Build history of the part. All positions in model axes, mm. Face numbers are marked on the shaded views. A direction names the side the tool comes from. Give positions to 0.01 mm unless a question says otherwise; leave off trailing zeros. Order: outer loops, then holes, each group sorted by start corner. A loop starts at its lowest first (then second) coordinate and runs counter-clockwise, first axis right, second up. Notation, with made-up numbers: (39.25, -22) - (70.25, -22) arc R15 ccw to (70.25, 3) - close; hole circle Ø3 at (86, -39). An arc over 180 degrees is marked (long way). Use a Markdown table: item, result.
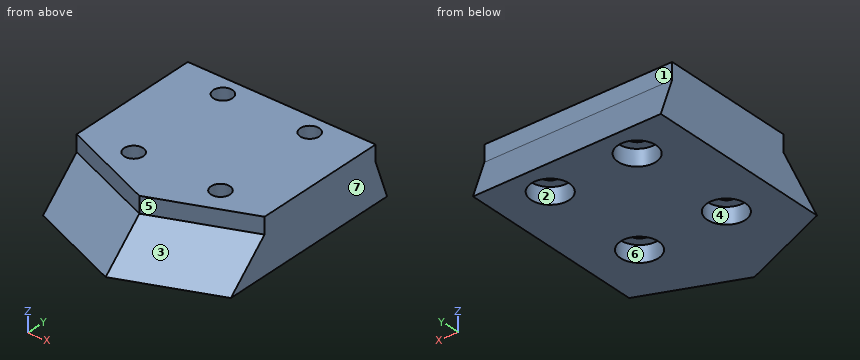
from build123d import *

# Parameters (mm, degrees)
ESBO_O1_W                = 34.6
ESBO_O1_H                = 26
RESSALTO_EXTRUS_O1_DEPTH = 7
ESBO_O10_W               = 34.6
ESBO_O10_H               = 2.5
RESSALTO_EXTRUS_O4_DEPTH = 7
CHANFRO1_SIZE            = 7
CHANFRO2_SIZE2           = 7
CHANFRO2_SIZE            = 2.54779164
RESSALTO_EXTRUS_O5_DEPTH = 3
ESBO_O11_R               = 1.75
CORTE_EXTRUS_O1_DEPTH    = 10
ESBO_O12_R               = 3.5
CORTE_EXTRUS_O2_DEPTH    = 3


with BuildPart() as part:
    # Esboço1 → Ressalto-extrusão1 (new body)
    with BuildSketch(Plane.XY):
        Rectangle(ESBO_O1_W, ESBO_O1_H)
    extrude(amount=RESSALTO_EXTRUS_O1_DEPTH)

    # Esboço10 → Ressalto-extrusão4 (add)
    with BuildSketch(Plane(origin=(0, 0, 0), x_dir=(-1, 0, 0), z_dir=(0, 0, -1))):
        Polygon((-17.3, -19.5), (0, -26.5), (17.3, -19.5), (17.3, -13), (-17.3, -13), align=None)
        with Locations((0, 14.25)):
            Rectangle(ESBO_O10_W, ESBO_O10_H)
    extrude(amount=-RESSALTO_EXTRUS_O4_DEPTH)

    # Chanfro1
    chanfro1_edges = [part.edges().sort_by_distance(p)[0] for p in [
        (8.65, -23, 7),
        (-8.65, -23, 7),
    ]]
    chamfer(chanfro1_edges, length=CHANFRO1_SIZE - 0.0001)  # a hair under: the kernel refuses the full size

    # Chanfro2
    chanfro2_edges = [part.edges().sort_by_distance(p)[0] for p in [
        (0, 15.5, 7),
    ]]
    chanfro2_side = [part.faces().sort_by_distance(p)[0] for p in [
        (0, 15.449044167, 7),
    ]]
    chamfer(chanfro2_edges, length=CHANFRO2_SIZE - 0.0001, length2=CHANFRO2_SIZE2 - 0.0001, reference=chanfro2_side[0])  # a hair under: the kernel refuses the full size

    # Esboço13 → Ressalto-extrusão5 (add)
    with BuildSketch(Plane.XY.offset(7)):
        Polygon((17.3, -11.948687565), (17.3, 12.95220836), (-17.3, 12.95220836), (-17.3, -11.948687565), (0, -18.948687565), align=None)
    extrude(amount=RESSALTO_EXTRUS_O5_DEPTH)

    # Esboço11 → Corte-extrusão1 (cut)
    with BuildSketch(Plane.XY.offset(10)):
        with Locations((8, 9.5)):
            Circle(ESBO_O11_R)
        with Locations((8, -10.5)):
            Circle(ESBO_O11_R)
        with Locations(Location((-8, -10.5, 0), (0, 0, 180))):
            Circle(ESBO_O11_R)
        with Locations(Location((-8, 9.5, 0), (0, 0, 180))):
            Circle(ESBO_O11_R)
    extrude(amount=-CORTE_EXTRUS_O1_DEPTH, mode=Mode.SUBTRACT)

    # Esboço12 → Corte-extrusão2 (cut)
    with BuildSketch(Plane(origin=(0, 0, 0), x_dir=(-1, 0, 0), z_dir=(0, 0, -1))):
        with Locations((-8, 9.5)):
            Circle(ESBO_O12_R)
        with Locations((8, 9.5)):
            Circle(ESBO_O12_R)
        with Locations((-8, -10.5)):
            Circle(ESBO_O12_R)
        with Locations((8, -10.5)):
            Circle(ESBO_O12_R)
    extrude(amount=-CORTE_EXTRUS_O2_DEPTH, mode=Mode.SUBTRACT)


solid = part.part
1) Wall check: line 1 (X direction, y = 9, z = 1.5); line 2 (Y direction, x = 9, z = 1); line 3 (X direction, y = 6.5, z = 0.75). Give the ranges that are in metal, low to high. Write a range as from..to.
Computed:
| item | result |
|---|---|
| line 1 | x = -17.3..-11.46, -4.54..4.54, 11.46..17.3 |
| line 2 | y = -21.78..-13.85, -7.15..6.15, 12.85..15.14 |
| line 3 | x = -17.3..-9.8, -6.2..6.2, 9.8..17.3 |
2) Slice it at B-B (z = 7.75). Write the cut outline in (x, y), and give its area (3 significant figures).
Computed:
| item | result |
|---|---|
| outline | (-17.3, -11.95) - (0, -18.95) - (17.3, -11.95) - (17.3, 12.95) - (-17.3, 12.95) - close; hole circle Ø3.5 at (-8, -10.5); hole circle Ø3.5 at (-8, 9.5); hole circle Ø3.5 at (8, -10.5); hole circle Ø3.5 at (8, 9.5) |
| area | 944 mm² |
3) Slice it at A-A (y = -10.5). Write the cut outline in (x, z), and give its area (3 significant figures).
Computed:
| item | result |
|---|---|
| outline | (-17.3, 0) - (-11.5, 0) - (-11.5, 3) - (-9.75, 3) - (-9.75, 10) - (-17.3, 10) - close; (-6.25, 3) - (-4.5, 3) - (-4.5, 0) - (4.5, 0) - (4.5, 3) - (6.25, 3) - (6.25, 10) - (-6.25, 10) - close; (9.75, 3) - (11.5, 3) - (11.5, 0) - (17.3, 0) - (17.3, 10) - (9.75, 10) - close |
| area | 255 mm² |
4) Tool access for the marked faces 5, 6 and 7: list every direction of +Z, -Z, +X, -X, +Y, -Y with a clear straight run to the whole face (end or side of a thin tool).
Computed:
| item | result |
|---|---|
| face 5 | +Z, +X, -Y |
| face 6 | -Z |
| face 7 | +Z, -Z, +X, +Y, -Y |
5) Pin check, flat tips, straight feed: P1, Ø6, axis at x = -1, z = 7.5, coming from the +Y side; P2, Ø6.5, axis at x = -8, y = -10.5, coming from the +Z side; P3, Ø6, axis at x = 3.5, z = 8, coming from the +Y side; P4, Ø2, axis at x = 8.5, y = -9, coming from the -Z side. Stop position of each tip, or through.
Computed:
| item | result |
|---|---|
| P1 | stops at y = 13.86 |
| P2 | stops at z = 10 |
| P3 | stops at y = 13.68 |
| P4 | stops at z = 3 |
6) Two-plate mould, pull along X, no slides. Class the marked faces 1, 2, 3 and 4: +X half, -X half, draft (parallel to the pull), parting line (faces both ways), or undercut.
Computed:
| item | result |
|---|---|
| face 1 | draft |
| face 2 | undercut |
| face 3 | +X half |
| face 4 | undercut |
7) Slice it at C-C (x = -8). State how many separate pieces and enclosed holes the cut face has, and give its area (3 significant figures).
Computed:
| item | result |
|---|---|
| separate pieces | 3 |
| enclosed holes | 0 |
| area | 231 mm² |
